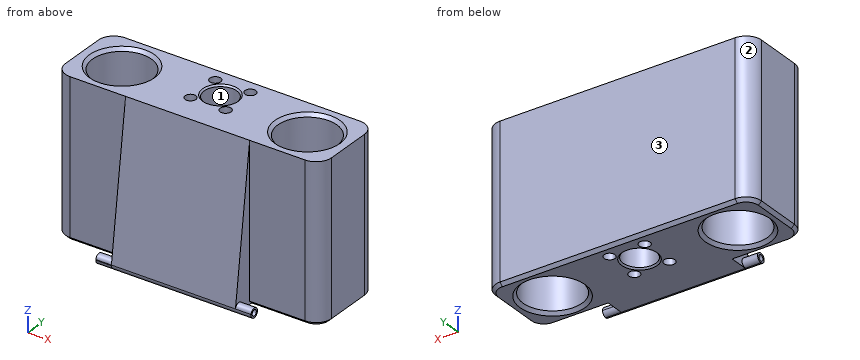
from build123d import *
from build123d import SkipClean  # not in build123d's __all__

# Parameters (mm, degrees)
F0_W      = 85.7687139645
F0_H      = 25
F0_R      = 9.5
F0_R_2    = 5.25
F1_DEPTH  = 50
F3_R      = 0.95
F4_DEPTH  = 20
F5_R      = 0.95
F6_DEPTH  = 5
F7_R      = 0.95
F8_DEPTH  = 5
F9_R      = 1.75
F10_DEPTH = 50
F11_R     = 5
F12_SIZE  = 1
F13_SIZE  = 0.5
F14_SIZE  = 1


# Not quite as in the source:
# - after a boolean that leaves OpenCascade's solid faulty, fix() repairs it


with BuildPart() as f1:
    # F0 (on Top) → F1 (new body)
    with BuildSketch(Plane.XY):
        with Locations((0, 168.5)):
            Rectangle(F0_W, F0_H)
        with Locations((-29.8843569823, 168.3684210526)):
            Circle(F0_R, mode=Mode.SUBTRACT)
        with Locations((29.8843569823, 168.3684210526)):
            Circle(F0_R, mode=Mode.SUBTRACT)
        with Locations((0, 171)):
            Circle(F0_R_2, mode=Mode.SUBTRACT)
    extrude(amount=F1_DEPTH)

    # F3 (on mid) → F4 (join, symmetric)
    with BuildSketch(Plane.YZ):
        with BuildLine():
            Line((156, 50), (149.5133467482, 1.6996549744))
            ThreePointArc((149.5133467482, 1.6996549744), (149.8709556117, 0.5124480929), (151, 0))
            Line((151, 0), (156, 0))
            Line((156, 0), (156, 50))
        make_face()
        with Locations((151, 1.5)):
            Circle(F3_R, mode=Mode.SUBTRACT)
    extrude(amount=F4_DEPTH, both=True)

    # F5 (on face) → F6 (join)
    with BuildSketch(Plane.YZ.offset(20)):
        with BuildLine():
            ThreePointArc((151, 0), (152.0606601718, 0.4393398282), (152.5, 1.5))
            ThreePointArc((152.5, 1.5), (151.100050293, 2.9966595935), (149.5133467482, 1.6996549744))
            ThreePointArc((149.5133467482, 1.6996549744), (149.8709556117, 0.5124480929), (151, 0))
        make_face()
        with Locations((151, 1.5)):
            Circle(F5_R, mode=Mode.SUBTRACT)
    extrude(amount=F6_DEPTH)

    # F7 (on face) → F8 (join)
    with BuildSketch(Plane(origin=(-20, 0, 0), x_dir=(0, -1, 0), z_dir=(-1, 0, 0))):
        with BuildLine():
            ThreePointArc((-151, 0), (-149.9393398282, 0.4393398282), (-149.5, 1.5))
            ThreePointArc((-149.5, 1.5), (-149.5033404065, 1.600050293), (-149.5133467482, 1.6996549744))
            ThreePointArc((-149.5133467482, 1.6996549744), (-152.1290443883, 2.4875519071), (-151, 0))
        make_face()
        with Locations((-151, 1.5)):
            Circle(F7_R, mode=Mode.SUBTRACT)
    with SkipClean():  # cleaning this boolean's faces spoils the solid; the shape is the same uncleaned
        extrude(amount=F8_DEPTH)

    # F9 (on face) → F10 (cut, through all)
    with BuildSketch(Plane.XY.offset(50)):
        with Locations((5.6568542495, 176.6568542495)):
            Circle(F9_R)
        with Locations((-5.6568542495, 176.6568542495)):
            Circle(F9_R)
        with Locations((-5.6568542495, 165.3431457505)):
            Circle(F9_R)
        with Locations((5.6568542495, 165.3431457505)):
            Circle(F9_R)
    extrude(amount=-F10_DEPTH, mode=Mode.SUBTRACT)

    add(f1.part.fix(), mode=Mode.REPLACE)

    # F11
    f11_edges = [f1.edges().sort_by_distance(p)[0] for p in [
        (42.884357, 156, 25),
        (42.884357, 181, 25),
        (-42.884357, 181, 25),
        (-42.884357, 156, 25),
    ]]
    fillet(f11_edges, radius=F11_R)

    # F12
    f12_edges = [f1.edges().sort_by_distance(p)[0] for p in [
        (20.384357, 168.368421, 50),
        (-39.384357, 168.368421, 50),
        (20.384357, 168.368421, 0),
        (-39.384357, 168.368421, 0),
    ]]
    chamfer(f12_edges, length=F12_SIZE)

    # F13
    f13_edges = [f1.edges().sort_by_distance(p)[0] for p in [
        (-5.25, 171, 50),
        (-5.25, 171, 0),
    ]]
    chamfer(f13_edges, length=F13_SIZE)

    # F14
    f14_edges = [f1.edges().sort_by_distance(p)[0] for p in [
        (-28.942178, 156, 0),
        (-41.419891, 157.464466, 0),
        (42.884357, 168.5, 0),
        (41.419891, 157.464466, 0),
        (41.419891, 179.535534, 0),
        (28.942178, 156, 0),
        (0, 181, 0),
        (-41.419891, 179.535534, 0),
        (-42.884357, 168.5, 0),
    ]]
    chamfer(f14_edges, length=F14_SIZE)


solid = f1.part
Work out the finished part from the listing and answer in its coordinate system (mm). Face numbers are marked on the shaded views. Round coordinates to 2 decimals unless told otherwise and drop trailing zeros. Order: outer loops, then holes, each group sorted by start corner. A loop starts at its lowest first (then second) coordinate and runs counter-clockwise, first axis right, second up. Notation, with made-up numbers: M 2.25,83.25 L 30.25,83.25 A19 ccw 30.25,89.25 Z; hole C 77,-6 d10. An arc over 180 degrees is marked long. Put each result on its own line as item: value. Start each with the question number.
Q1. Flat-ended cylindrical pins translate along their axes: pin 1 (6.5 mm diameter, centred on x = 0, y = 171, fed in from -Z); pin 2 (2.5 mm diameter, centred on y = 151.5, z = 1.5, fed in from -X); pin 3 (6 mm diameter, centred on y = 152, z = 26.5, fed in from -X); pin 4 (2 mm diameter, centred on y = 154, z = 36, fed in from +X). Find the tip coordinate at first contact, or state that the pin passes through.
Q2. For a pull along X with two mould halves and no side action, classify the marked faces 1, 2 and 3 as pulls with the +X half, pulls with the -X half, needs draft (parallel to the pull), parting line crosses it, or undercut.
Q3. Section B-B, the plane z = 32.5 is taken. Write down the section's boundary in (x, y), and give its area (3 significant figures).
Q4. Section A-A, the plane x = -16 is taken. Write down the section's boundary in (y, z), and give its area (3 significant figures).
Q5. Straight lines are drawn through the part: L1, parallel to Z at x = -23.5, y = 151; L2, parallel to X at y = 163, z = 35.5; L3, parallel to X at y = 164, z = 26.5. For each, find the intervals that lie inside material, in ascending order. Write a range as [from, to].
Q6. Section C-C, the plane z = 21.5 is taken. Write down the section's boundary in (x, y).
Q7. Section D-D, the plane y = 170 is taken. Give the number of separate pieces and of enclosed holes in the cut face, and give its area (3 significant figures).
Findings below:
1. pin 1: passes through
1. pin 2: stops at x = -25
1. pin 3: stops at x = -20
1. pin 4: stops at x = 20
2. face 1: undercut
2. face 2: pulls with the -X half
2. face 3: needs draft
3. outline: M -42.88,161 A5 ccw -37.88,156 L -20,156 L -20,153.65 L 20,153.65 L 20,156 L 37.88,156 A5 ccw 42.88,161 L 42.88,176 A5 ccw 37.88,181 L -37.88,181 A5 ccw -42.88,176 Z; hole C -29.88,168.37 d19; hole C -5.66,165.34 d3.5; hole C -5.66,176.66 d3.5; hole C 0,171 d10.5; hole C 5.66,165.34 d3.5; hole C 5.66,176.66 d3.5; hole C 29.88,168.37 d19
3. area: 1,520 mm^2
4. outline: M 149.51,1.7 A1.5 ccw 151,0 L 180,0 L 181,1 L 181,50 L 156,50 Z; hole C 151,1.5 d1.9
4. area: 1,410 mm^2
5. L1: z = [0, 0.55], [2.45, 3]
5. L2: x = [-42.88, -37.72], [-22.05, 22.05], [37.72, 42.88]
5. L3: x = [-42.88, -38.32], [-21.45, -6.78], [-4.54, 4.54], [6.78, 21.45], [38.32, 42.88]
6. outline: M -42.88,161 A5 ccw -37.88,156 L -20,156 L -20,152.17 L 20,152.17 L 20,156 L 37.88,156 A5 ccw 42.88,161 L 42.88,176 A5 ccw 37.88,181 L -37.88,181 A5 ccw -42.88,176 Z; hole C -29.88,168.37 d19; hole C -5.66,165.34 d3.5; hole C -5.66,176.66 d3.5; hole C 0,171 d10.5; hole C 5.66,165.34 d3.5; hole C 5.66,176.66 d3.5; hole C 29.88,168.37 d19
7. separate pieces: 4
7. enclosed holes: 0
7. area: 1,900 mm^2
